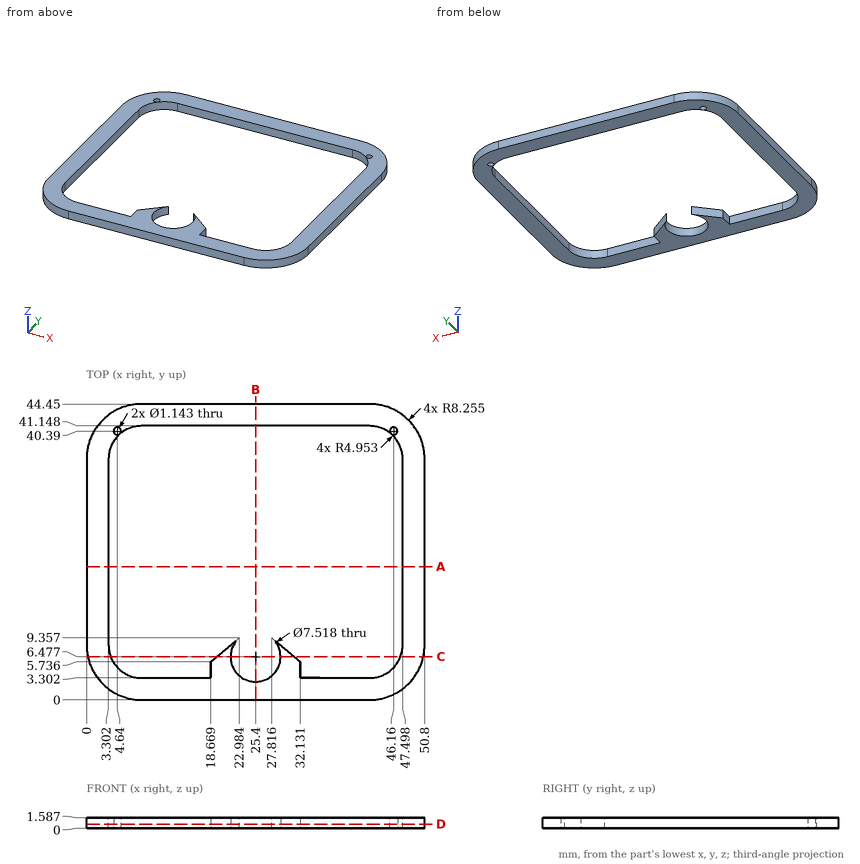
For this review, use the dimensioned drawing (mm, ordinates from the lowest corner) and the shaded views. Round coordinates to 2 decimals unless told otherwise and drop trailing zeros. Order: outer loops, then holes, each group sorted by start corner. A loop starts at its lowest first (then second) coordinate and runs counter-clockwise, first axis right, second up. Notation, with made-up numbers: (2, 38) -> (13, 38) arc R22 cw to (13, 46) -> close; hole circle Ø8 at (71, 24.5). An arc over 180 degrees is marked (long way). Write item = value, one per line. Start each with the question number.
Item 1: Consider section C-C on y = 6.5. Write out the cut boundary in (x, z).
Item 2: For line 1 along Y through (x, z) = (25.4, 0.9); line 2 along X through (y, z) = (15, 1.2); line 3 along Y through (x, z) = (9, 0.95), list the stretches that pass through material, from the lowest coordinate up.
Item 3: Consider section D-D on z = 0.65. Count the separate pieces of the cut face and the enclosed holes in it.
Item 4: Consider section B-B on x = 25.4. Write out the cut boundary in (y, z).
Item 5: Clearance check with flat-ended pins moving along their axes: pin 1 Ø1.5 at (x, y) = (32, 9) entering from -Z; pin 2 Ø0.8 at (y, z) = (4.5, 1) entering from -X; pin 3 Ø0.8 at (y, z) = (4, 1) entering from +X (1 decimal); pin 4 Ø0.5 at (y, z) = (26, 0.5) entering from -X. State where each tip first meets the part, or that it passes through.
Item 6: Consider section A-A on y = 20. Write out the cut boundary in (x, z), plus the area to 3 significant figures.
Conclusion:
q1.outline = (0.19, 0) -> (3.62, 0) -> (3.62, 1.59) -> (0.19, 1.59) -> close; (19.58, 0) -> (21.64, 0) -> (21.64, 1.59) -> (19.58, 1.59) -> close; (29.16, 0) -> (31.22, 0) -> (31.22, 1.59) -> (29.16, 1.59) -> close; (47.18, 0) -> (50.61, 0) -> (50.61, 1.59) -> (47.18, 1.59) -> close
q2.line_1 = 0 to 2.72, 41.15 to 44.45
q2.line_2 = 0 to 3.3, 47.5 to 50.8
q2.line_3 = 0 to 3.3, 41.15 to 44.45
q3.separate_pieces = 1
q3.enclosed_holes = 3
q4.outline = (0, 0) -> (2.72, 0) -> (2.72, 1.59) -> (0, 1.59) -> close; (41.15, 0) -> (44.45, 0) -> (44.45, 1.59) -> (41.15, 1.59) -> close
q5.pin_1 = through
q5.pin_2 = 0.71
q5.pin_3 = 49.8
q5.pin_4 = 0
q6.outline = (0, 0) -> (3.3, 0) -> (3.3, 1.59) -> (0, 1.59) -> close; (47.5, 0) -> (50.8, 0) -> (50.8, 1.59) -> (47.5, 1.59) -> close
q6.area = 10.5 mm2
